Source: three-view drawing plus pictorial views. Frame: mm from the lowest corner of the part. Give positions to 0.01 mm unless a question says otherwise; leave off trailing zeros. Write each loop counter-clockwise with the first axis right and the second up, starting at its lowest first coordinate (ties: lowest second). Pieces come first, ordered by that corner, then holes.
Q1. Pin query (flat end, axial travel): pin 1 (0.8 mm diameter, centred on y = 61.5, z = 1, fed in from +X). Return the tip coordinate at first contact, or that it passes through.
Q2. Cut plane D-D on x = 16. Return the cut outline in (y, z).
Q3. Cut plane B-B on z = 1.85. Return the cut outline in (x, y) (1 decimal).
Q4. Cut plane A-A on x = 35. Return the cut outline in (y, z) (1 decimal), plus the area to 3 significant figures.
Q5. Line query: L1, parallel to Y at x = 36.5, z = 2.3 (1 decimal); L2, parallel to X at y = 61, z = 1.3 (1 decimal); L3, parallel to X at y = 34, z = 0.85 (1 decimal). Output: solid intervals per line, ascending.
Q6. Cut plane C-C on y = 9.5. Return the cut outline in (x, z), plus the area to 3 significant figures.
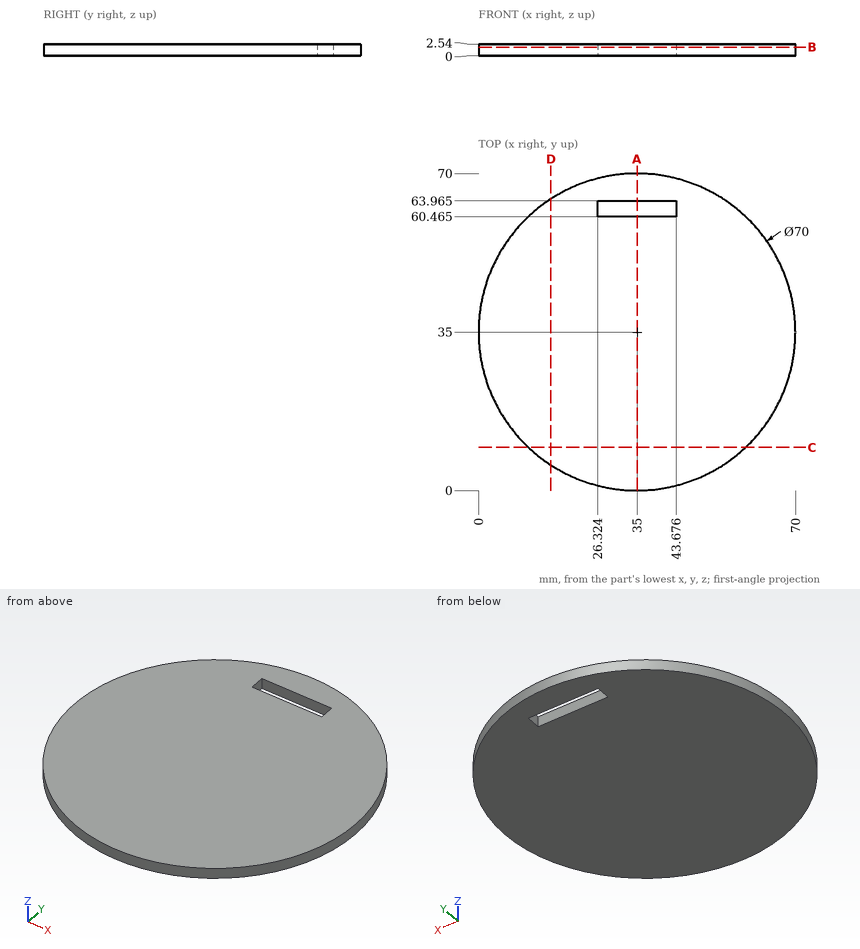
Data:
1. pin 1: stops at x = 58.32
2. outline: (5.61, 0) - (64.39, 0) - (64.39, 2.54) - (5.61, 2.54) - close
3. outline: circle Ø70 at (35, 35); hole (26.3, 60.5) - (43.7, 60.5) - (43.7, 64) - (26.3, 64) - close
4. outline: (0, 0) - (60.5, 0) - (60.5, 2.5) - (0, 2.5) - close; (64, 0) - (70, 0) - (70, 2.5) - (64, 2.5) - close
4. area: 169 mm2
5. L1: y = 0 to 60.5, 64 to 70
5. L2: x = 11.6 to 26.3, 43.7 to 58.4
5. L3: x = 0 to 70
6. outline: (11.03, 0) - (58.97, 0) - (58.97, 2.54) - (11.03, 2.54) - close
6. area: 122 mm2
